Build history of the part. All positions in model axes, mm. A direction names the side the tool comes from. Give positions to 0.01 mm unless a question says otherwise; leave off trailing zeros. Order: outer loops, then holes, each group sorted by start corner. A loop starts at its lowest first (then second) coordinate and runs counter-clockwise, first axis right, second up. Notation, with made-up numbers: M 8,-17.5 L 59,-17.5 A25 cw 59,21.5 Z; hole C 32.25,45 d11. An arc over 180 degrees is marked long. Use CSV: the item, a comma, the result in double quotes. Start each with the question number.
Item 1: Band-saw the part on D-D on y = 2. Write the cut outline in (x, z).
Item 2: Which spindle directions (+Z, -Z, +X, -X, +Y, -Y) get a long thin tool onto all of the face, cutting with end or side? Do faces 5 (the cylindrical face through (68.965, -9.769, 20.193)), 6 (the flat face through (48, -10, 10)), 7 (the flat face through (50.255, 24, -11)), 8 (the flat face through (33, 13, 3)), 9 (the flat face through (33, 13, -3)). Say none if no direction does.
Item 3: Pin check, flat tips, straight feed: P1, Ø8, axis at x = 51, y = -8.5, coming from the -Z side; P2, Ø8, axis at y = -10.5, z = 2.5, coming from the -X side; P3, Ø4, axis at x = 42, y = 6.5, coming from the -Z side; P4, Ø0.6, axis at y = 23.5, z = -11, coming from the +X side. Stop position of each tip, or through.
Item 4: Band-saw the part on C-C on x = 65.5. Write the cut outline in (y, z), plus the area to 3 significant figures.
Item 5: Wall check: line 1 along Y through (x, z) = (41, -18); line 2 along Z through (x, y) = (27, 10.5); line 3 along X through (y, z) = (23, 0). Give the ranges that are in metal, low to high.
Item 6: Two-plate mould, pull along X, no slides. Class faces 1 (the flat face through (43, 0, -4)), 2 (the conical face through (37.481, 24.865, -24.872)), 3 (the cylindrical face through (34.86, -9.17, 12.59)), 4 (the cylindrical face through (57.743, 12.886, 7.105)): pulls with the +X half, pulls with the -X half, needs draft (parallel to the pull), parting line crosses it, or undercut.
Item 7: Band-saw the part on B-B on y = -10. Write the cut outline in (x, z).
Item 8: Band-saw the part on A-A on y = 12.5. Write the cut outline in (x, z), plus the area to 3 significant figures.
from build123d import *

# Parameters (mm, degrees)
SKETCH1_R                       = 2.5
BOSS_EXTRUDE1_DEPTH             = 25
SKETCH9_W                       = 45.48
SKETCH9_H                       = 45
BOSS_EXTRUDE4_DEPTH             = 15
CUT_EXTRUDE2_START              = -2.5
CUT_EXTRUDE2_DEPTH              = 19.5
SKETCH15_R                      = 2.5
BOSS_EXTRUDE5_DEPTH             = 25
CHAMFER1_SIZE                   = 10
CUT_EXTRUDE3_REACH              = 47.48
SKETCH16_W                      = 40
SKETCH16_H                      = 19.5
SKETCH17_W                      = 15.08
SKETCH17_H                      = 6
BOSS_EXTRUDE6_DEPTH             = 22
CBORE_FOR_M5_SBHCS1_D           = 5.5
CBORE_FOR_M5_SBHCS1_CBORE_D     = 10.5
CBORE_FOR_M5_SBHCS1_CBORE_DEPTH = 9.75
CHAMFER2_SIZE                   = 0.5


with BuildPart() as part:
    # Sketch1 → Boss-Extrude1 (new body)
    with BuildSketch(Plane(origin=(0, 0, 0), x_dir=(1, 0, 0), z_dir=(0, 1, 0))):
        Polygon((20.24, -10), (25.24, -10), (25.24, 10), (20.24, 10), (-20.24, 10), (-20.24, -10), align=None)
        Circle(SKETCH1_R, mode=Mode.SUBTRACT)
    extrude(amount=BOSS_EXTRUDE1_DEPTH)

    # Sketch9 → Boss-Extrude4 (add)
    with BuildSketch(Plane.XY.offset(10)):
        with Locations((2.5, 2.5)):
            Rectangle(SKETCH9_W, SKETCH9_H)
    extrude(amount=BOSS_EXTRUDE4_DEPTH)

    # Sketch10 → Cut-Extrude2 (cut)
    with BuildSketch(Plane(origin=(0, 25, 0), x_dir=(1, 0, 0), z_dir=(0, 1, 0)).offset(CUT_EXTRUDE2_START)):
        with BuildLine():
            Line((10.16, 0), (10.16, 10))
            Line((10.16, 10), (-10.16, 10))
            Line((-10.16, 10), (-10.16, 0))
            ThreePointArc((-10.16, 0), (0, -10.16), (10.16, 0))
        make_face()
    extrude(amount=-CUT_EXTRUDE2_DEPTH, mode=Mode.SUBTRACT)

    # Sketch15 → Boss-Extrude5 (add)
    with BuildSketch(Plane(origin=(0, 25, 0), x_dir=(1, 0, 0), z_dir=(0, 1, 0))):
        with BuildLine():
            Line((25.24, 10), (25.24, 12.732395665))
            ThreePointArc((25.24, 12.732395665), (12.732395665, 25.24), (0.224791329, 12.732395665))
            Line((0.224791329, 12.732395665), (0.224791329, 10))
            Line((0.224791329, 10), (25.24, 10))
        make_face()
        with Locations((12.732395665, 12.732395665)):
            Circle(SKETCH15_R, mode=Mode.SUBTRACT)
    extrude(amount=-BOSS_EXTRUDE5_DEPTH)

    # Chamfer1
    chamfer1_edges = [part.edges().sort_by_distance(p)[0] for p in [
        (2.5, 25, 25),
    ]]
    chamfer(chamfer1_edges, length=CHAMFER1_SIZE)

    # Sketch16 → Cut-Extrude3 (cut, up to next)
    with BuildSketch(Plane(origin=(25.24, 0, 0), x_dir=(0, 0, -1), z_dir=(1, 0, 0)), mode=Mode.PRIVATE) as cut_extrude3_sk1:
        with Locations((9.84, 12.75)):
            Rectangle(SKETCH16_W, SKETCH16_H)
    cut_extrude3_tool1 = extrude(cut_extrude3_sk1.sketch, amount=-CUT_EXTRUDE3_REACH, mode=Mode.PRIVATE) & part.part
    add(cut_extrude3_tool1.solids().sort_by_distance((25.24, 12.75, -9.84))[0], mode=Mode.SUBTRACT)

    # Sketch17 → Boss-Extrude6 (add)
    with BuildSketch(Plane(origin=(0, 25, 0), x_dir=(1, 0, 0), z_dir=(0, 1, 0))):
        with Locations((17.7, 0)):
            Rectangle(SKETCH17_W, SKETCH17_H)
    extrude(amount=-BOSS_EXTRUDE6_DEPTH)

    # CBORE for M5 SBHCS1 (through all)
    with Locations(Plane.XY.offset(25)):
        with Locations((-13.24, -10), (18.24, -10)):
            CounterBoreHole(CBORE_FOR_M5_SBHCS1_D / 2, CBORE_FOR_M5_SBHCS1_CBORE_D / 2, CBORE_FOR_M5_SBHCS1_CBORE_DEPTH)


with BuildPart() as body_2:
    # Mirror1: mirrored copy
    add(part.part.mirror(Plane(origin=(25.24, 25, 10), x_dir=(0, 0, 1), z_dir=(-1, 0, 0))))

    # Chamfer2
    chamfer2_edges = [body_2.edges().sort_by_distance(p)[0] for p in [
        (70.72, 25, 2.5),
        (47.98, -20, 25),
        (25.24, -2.5, 25),
        (60.487604335, 25, -10),
        (37.747604335, 25, -25.24),
        (50.255208671, 25, -11.366197832),
        (70.72, -2.5, 25),
        (70.72, 20, 20),
        (25.24, 25, 1.133802168),
        (25.24, 20, 20),
    ]]
    chamfer(chamfer2_edges, length=CHAMFER2_SIZE)


solid = body_2.part
Model answer:
1,outline,"M 25.24,-12.73 A12.51 ccw 50.26,-12.73 L 50.26,-10 L 70.72,-10 L 70.72,24.5 L 70.22,25 L 25.74,25 L 25.24,24.5 Z; hole C 37.75,-12.73 d5; hole C 50.48,0 d5"
2,face 5,"+Z"
2,face 6,"-Z, +X, -X, -Y"
2,face 7,"-Z, +X, +Y, -Y"
2,face 8,"-X"
2,face 9,"-Z, -X"
3,P1,"stops at z = 10"
3,P2,"passes through"
3,P3,"stops at z = -3"
3,P4,"stops at x = 50.26"
4,outline,"M -20,10 L -12.1,10 L -12.1,15.25 L -14.94,15.25 L -14.94,25 L -19.5,25 L -20,24.5 Z; M -7.9,10 L 0,10 L 0,-10 L 24.5,-10 L 25,-9.5 L 25,15 L 15,25 L -5.06,25 L -5.06,15.25 L -7.9,15.25 Z"
4,area,"1,010 mm^2"
5,line 1,"y = 0 to 3, 22.5 to 25"
5,line 2,"z = -3 to 3, 10.16 to 25"
5,line 3,"x = 25.24 to 47.98, 52.98 to 70.72"
6,face 1,"needs draft"
6,face 2,"parting line crosses it"
6,face 3,"undercut"
6,face 4,"undercut"
7,outline,"M 25.24,10 L 29.49,10 L 29.49,15.25 L 26.99,15.25 L 26.99,25 L 25.74,25 L 25.24,24.5 Z; M 34.99,10 L 60.97,10 L 60.97,15.25 L 58.47,15.25 L 58.47,25 L 37.49,25 L 37.49,15.25 L 34.99,15.25 Z; M 66.47,10 L 70.72,10 L 70.72,24.5 L 70.22,25 L 68.97,25 L 68.97,15.25 L 66.47,15.25 Z"
8,outline,"M 25.24,-3 L 40.32,-3 L 40.32,3 L 25.24,3 Z; M 25.24,10.16 L 50.48,10.16 A10.16 cw 60.64,0 L 60.64,-10 L 70.72,-10 L 70.72,24.5 L 70.22,25 L 25.74,25 L 25.24,24.5 Z"
8,area,"991 mm^2"
